Read the model definition and answer for the solid it produces. Units are mm, in the model's axes. Give positions to 0.01 mm unless a question says otherwise; leave off trailing zeros. Loops run counter-clockwise (first coordinate to the right, second up) from the corner with the lowest first, then second, coordinate; pieces in that order, holes last. Notation, with made-up numbers: (42.5, 29) - (55.5, 29) arc R31 ccw to (55.5, 55) - close; hole circle Ø9 at (-7.5, 62). An arc over 180 degrees is marked (long way). Write item = value, one per line.
```python
from build123d import *

# Parameters (mm, degrees)
CORTE_EXTRUS_O1_DEPTH      = 25.768326548
CORTE_EXTRUS_O1_DEPTH_BACK = 25.768326548
ESBO_O2_W                  = 15
ESBO_O2_H                  = 30
ESBO_O3_R                  = 8
CORTE_EXTRUS_O2_DEPTH      = 33.000312498
FILETE1_R                  = 0.6
SCALE1_SCALE               = 0.5


with BuildPart() as part:
    # Esboço1 → Revolução1 (revolve)
    with BuildSketch(Plane.XY):
        with BuildLine():
            Line((0, -14.3), (0, 14.3))
            ThreePointArc((0, 14.3), (14.3, 0), (0, -14.3))
        make_face()
    revolve(axis=Axis((0, -14.3, 0), (0, 1, 0)))

    # Esboço2 → Corte-extrusão1 (cut, two sides: drawn at the far end of the back side and taken through both)
    with BuildSketch(Plane(origin=(0, 0, 0), x_dir=(0, 0, -1), z_dir=(1, 0, 0)).offset(-CORTE_EXTRUS_O1_DEPTH_BACK)):
        with Locations((-18, 0)):
            Rectangle(ESBO_O2_W, ESBO_O2_H)
        with Locations((18, 0)):
            Rectangle(ESBO_O2_W, ESBO_O2_H)
    extrude(amount=CORTE_EXTRUS_O1_DEPTH + CORTE_EXTRUS_O1_DEPTH_BACK, mode=Mode.SUBTRACT)

    # Esboço3 → Corte-extrusão2 (cut, through all)
    with BuildSketch(Plane.XY.offset(10.5)):
        Circle(ESBO_O3_R)
    extrude(amount=-CORTE_EXTRUS_O2_DEPTH, mode=Mode.SUBTRACT)

    # Filete1
    filete1_edges = [part.edges().sort_by_distance(p)[0] for p in [
        (0, 9.70772888, -10.5),
        (-8, 0, -10.5),
        (-8, 0, 10.5),
        (0, 9.70772888, 10.5),
    ]]
    fillet(filete1_edges, radius=FILETE1_R)


with BuildPart() as part_1:
    # Scale1: scaled about (-1.207e-06, 2.588e-06, 0)
    add(part.part.scale(SCALE1_SCALE).moved(Location((-6.04e-07, 1.294e-06, 0))))


solid = part_1.part
```
1) Find the intervals of material crossed by probe 1 along X at (y, z) = (1, -2.5); probe 2 along X at (y, z) = (-3, 0.5); probe 3 along Y at (x, z) = (0, -0.75), in increasing order.
Output:
probe_1 = -6.62 to -3.87, 3.87 to 6.62
probe_2 = -6.47 to -2.65, 2.65 to 6.47
probe_3 = -7.11 to -4, 4 to 7.11
2) A cutting plane is placed at A-A on z = -2. Determine the outline of the cut face in (x, y).
Output:
outline = circle Ø13.73 at (0, 0); hole circle Ø8 at (0, 0)
3) Each of these flat-tipped pins is pushed along its axis until it touches: P1, Ø4, axis at y = 4, z = 4, coming from the +X side; P2, Ø3, axis at y = 4, z = -2, coming from the +X side; P3, Ø2, axis at y = -2, z = -1.5, coming from the -X side; P4, Ø5, axis at y = 2, z = 0.5, coming from the +X side. Where does it stop, or does it pass through?
Output:
P1 = 6.14
P2 = 6.5
P3 = -6.99
P4 = 7.15
4) The mould has two halves that part along X. Classify faces 1 (the face through (-0.867, -3.905, 0.069)), 2 (the face through (2, -4, 5.25)): pulls with the +X half, pulls with the -X half, needs draft (parallel to the pull), parting line crosses it, or undercut.
Output:
face_1 = undercut
face_2 = needs draft
